```python
from build123d import *

# Parameters (mm, degrees)
SKETCH1_W                = 400
SKETCH1_H                = 700
BOSS_EXTRUDE1_DEPTH      = 10
BOSS_EXTRUDE2_DEPTH      = 200
BOSS_EXTRUDE2_DEPTH_BACK = 200
CUT_EXTRUDE3_DEPTH       = 20
CUT_EXTRUDE3_DEPTH_BACK  = 20
CUT_EXTRUDE4_DEPTH       = 20
CUT_EXTRUDE4_DEPTH_BACK  = 20
CUT_EXTRUDE5_DEPTH       = 20
CUT_EXTRUDE5_DEPTH_BACK  = 20
SHELL3_START             = -189.5
SHELL3_DEPTH             = 379
SHELL3_START_2           = -124.5
SHELL3_2_DEPTH           = 94
SHELL3_START_3           = 30.5
SHELL3_3_DEPTH           = 94
SHELL3_4_DEPTH           = 4
SHELL3_START_4           = 185.5
SHELL3_5_DEPTH           = 4
SHELL3_START_5           = -30.5
SHELL3_6_DEPTH           = 61
FILLET1_R                = 100


# Read off the part's stored shape, not the designer's step: Shell3
with BuildPart() as part:
    # Sketch1 → Boss-Extrude1 (new body)
    with BuildSketch(Plane(origin=(0, 0, 0), x_dir=(1, 0, 0), z_dir=(0, 1, 0))):
        with Locations((0, 350)):
            Rectangle(SKETCH1_W, SKETCH1_H)
    extrude(amount=BOSS_EXTRUDE1_DEPTH)

    # Sketch2 → Boss-Extrude2 (add, two sides: drawn at the far end of the back side and taken through both)
    with BuildSketch(Plane(origin=(0, 0, 0), x_dir=(0, 0, -1), z_dir=(1, 0, 0)).offset(-BOSS_EXTRUDE2_DEPTH_BACK)):
        Polygon((0, 0), (0, 24.464411704), (101.405231438, 51.629278733), (207.601036066, 80.077464993), (207.601036066, 0), align=None)
    extrude(amount=BOSS_EXTRUDE2_DEPTH + BOSS_EXTRUDE2_DEPTH_BACK)

    # Sketch5 → Cut-Extrude3 (cut, two sides: drawn at the far end of the back side and taken through both)
    with BuildSketch(Plane(origin=(0, 0, 0), x_dir=(0, 0, -1), z_dir=(1, 0, 0)).offset(-CUT_EXTRUDE3_DEPTH_BACK)):
        with BuildLine():
            Line((207.651134237, 88.230641516), (207.651134237, 10))
            ThreePointArc((207.651134237, 10), (195.644591457, 43.3333125), (173.411266827, 70.918563406))
            Line((173.411266827, 70.918563406), (207.651134237, 88.230641516))
        make_face()
    extrude(amount=CUT_EXTRUDE3_DEPTH + CUT_EXTRUDE3_DEPTH_BACK, mode=Mode.SUBTRACT)

    # Sketch7 → Cut-Extrude4 (cut, two sides: drawn at the far end of the back side and taken through both)
    with BuildSketch(Plane(origin=(155, 0, 0), x_dir=(0, 0, -1), z_dir=(1, 0, 0)).offset(-CUT_EXTRUDE4_DEPTH_BACK)):
        with BuildLine():
            Line((207.601036066, 80.077464993), (207.601036066, 10))
            ThreePointArc((207.601036066, 10), (195.617643187, 43.328041458), (173.411266827, 70.918563406))
            Line((173.411266827, 70.918563406), (164.696313807, 94.748714882))
            Line((164.696313807, 94.748714882), (211.114914406, 101.759857681))
            Line((211.114914406, 101.759857681), (207.601036066, 80.077464993))
        make_face()
    extrude(amount=CUT_EXTRUDE4_DEPTH + CUT_EXTRUDE4_DEPTH_BACK, mode=Mode.SUBTRACT)

    # Sketch8 → Cut-Extrude5 (cut, two sides: drawn at the far end of the back side and taken through both)
    with BuildSketch(Plane(origin=(-155, 0, 0), x_dir=(0, 0, -1), z_dir=(1, 0, 0)).offset(-CUT_EXTRUDE5_DEPTH_BACK)):
        with BuildLine():
            Line((207.601036066, 10), (207.601036066, 80.077464993))
            Line((207.601036066, 80.077464993), (173.411266827, 70.918563406))
            ThreePointArc((173.411266827, 70.918563406), (195.617643187, 43.328041458), (207.601036066, 10))
        make_face()
    extrude(amount=CUT_EXTRUDE5_DEPTH + CUT_EXTRUDE5_DEPTH_BACK, mode=Mode.SUBTRACT)

    # Shell3 outline → Shell3 (cut)
    with BuildSketch(Plane.YZ.offset(SHELL3_START)):
        with BuildLine():
            Line((10.5, -10.5), (10.5, -196.809675626))
            ThreePointArc((10.5, -196.809675626), (36.812126695, -187.219283255), (59.262427205, -170.477489921))
            Line((59.262427205, -170.477489921), (16.406973107, -10.5))
            Line((16.406973107, -10.5), (10.5, -10.5))
        make_face()
    extrude(amount=SHELL3_DEPTH, mode=Mode.SUBTRACT)

    # Shell3 2 outline → Shell3 2 (cut)
    with BuildSketch(Plane.YZ.offset(SHELL3_START_2)):
        with BuildLine():
            Line((10.5, -207.601036066), (69.207241495, -207.601036066))
            Line((69.207241495, -207.601036066), (59.262427205, -170.477489921))
            ThreePointArc((59.262427205, -170.477489921), (36.812126695, -187.219283255), (10.5, -196.809675626))
            Line((10.5, -196.809675626), (10.5, -207.601036066))
        make_face()
    extrude(amount=SHELL3_2_DEPTH, mode=Mode.SUBTRACT)

    # Shell3 3 outline → Shell3 3 (cut)
    with BuildSketch(Plane.YZ.offset(SHELL3_START_3)):
        with BuildLine():
            Line((10.5, -207.601036066), (69.207241495, -207.601036066))
            Line((69.207241495, -207.601036066), (59.262427205, -170.477489921))
            ThreePointArc((59.262427205, -170.477489921), (36.812126695, -187.219283255), (10.5, -196.809675626))
            Line((10.5, -196.809675626), (10.5, -207.601036066))
        make_face()
    extrude(amount=SHELL3_3_DEPTH, mode=Mode.SUBTRACT)

    # Shell3 4 outline → Shell3 4 (cut)
    with BuildSketch(Plane.YZ.offset(SHELL3_START)):
        with BuildLine():
            Line((10.5, -197.101036066), (66.394456595, -197.101036066))
            Line((66.394456595, -197.101036066), (59.262427205, -170.477489921))
            ThreePointArc((59.262427205, -170.477489921), (36.812126695, -187.219283255), (10.5, -196.809675626))
            Line((10.5, -196.809675626), (10.5, -197.101036066))
        make_face()
    extrude(amount=SHELL3_4_DEPTH, mode=Mode.SUBTRACT)

    # Shell3 5 outline → Shell3 5 (cut)
    with BuildSketch(Plane.YZ.offset(SHELL3_START_4)):
        with BuildLine():
            Line((10.5, -197.101036066), (66.394456595, -197.101036066))
            Line((66.394456595, -197.101036066), (59.262427205, -170.477489921))
            ThreePointArc((59.262427205, -170.477489921), (36.812126695, -187.219283255), (10.5, -196.809675626))
            Line((10.5, -196.809675626), (10.5, -197.101036066))
        make_face()
    extrude(amount=SHELL3_5_DEPTH, mode=Mode.SUBTRACT)

    # Shell3 6 outline → Shell3 6 (cut)
    with BuildSketch(Plane.YZ.offset(SHELL3_START_5)):
        with BuildLine():
            Line((10.5, -196.809675626), (10.5, -196.858395835))
            ThreePointArc((10.5, -196.858395835), (36.816809355, -187.247785942), (59.263801063, -170.482618469))
            Line((59.263801063, -170.482618469), (59.262427205, -170.477489921))
            ThreePointArc((59.262427205, -170.477489921), (36.812126695, -187.219283255), (10.5, -196.809675626))
        make_face()
    extrude(amount=SHELL3_6_DEPTH, mode=Mode.SUBTRACT)

    # Fillet1
    # the kernel refuses this fillet: 100 mm, written as the material it takes off along each edge
    with BuildSketch(Plane(origin=(30.5, 10.5, -207.601036066), x_dir=(0, -1.0, -9.585505722497512e-10), z_dir=(1, 0, 0)), Plane(origin=(-124.5, 10.5, -207.601036066), x_dir=(0, -1.0, -9.585505722497512e-10), z_dir=(1, 0, 0))) as fillet1_piece_1:
        with BuildLine():
            CenterArc((99.99999999, -9.987492273), FILLET1_R, 174.26803198, 5.731967965)
            Line((-1e-08, -9.987492177), (0, 0))
            Line((0, 0), (0.5, 0))
        make_face()
    extrude(amount=94, mode=Mode.SUBTRACT)


solid = part.part
```
Can you work these out from the model? Positions are in its coordinate system, mm. A direction names the side the tool comes from. Round coordinates to 2 decimals unless told otherwise and drop trailing zeros. Order: outer loops, then holes, each group sorted by start corner. A loop starts at its lowest first (then second) coordinate and runs counter-clockwise, first axis right, second up. Notation, with made-up numbers: (21.5, -13.5) -> (26.5, -13.5) arc R23 ccw to (26.5, 23.5) -> close; hole circle Ø6 at (36.5, -5). An arc over 180 degrees is marked (long way). Return JSON: item names as keys, results as strings. Group by question number.
1. If we section it at D-D, the plane x = 164.5: Write out the boundary of the cut face in (y, z).
2. Which directions (+Z, -Z, +X, -X, +Y, -Y) give clear straight access to the entire face, cutting with the end or side of a thin tool? Please do faces 1 (the face through (-135, 58, -195)), 2 (the face through (-3, 0, -355)), 3 (the face through (-124.5, 46, -198)), 4 (the face through (185.5, 50, -190)), 5 (the face through (29, 56, -207.601)).
3. We'd pull the mould along X, two halves only. Please class faces 6 (the face through (-155.28, 43.762, -195.373)), 7 (the face through (-20, 53, -198)), 8 (the face through (187, 46, -207.601)), 9 (the face through (-200, 7, -219)): released by +X, released by -X, zero draft, split by the parting line, or undercut.
4. Will these pins go through, and if not, where does the flat tip stop? pin 1 (2 mm diameter, centred on x = -122, z = -539.5, fed in from +Y); pin 2 (12.5 mm diameter, centred on x = 189, y = 35.5, fed in from -Z); pin 3 (8 mm diameter, centred on x = -15.5, y = 40, fed in from -Z).
5. If we section it at C-C, the plane x = 56.5: Write out the boundary of the cut face in (y, z).
6. I need wall thicknesses on line 1 (Y direction, x = 13, z = -291); line 2 (Y direction, x = -98, z = -154.5); line 3 (Y direction, x = -106.5, z = -189). Which ranges of each line are inside material? Lowest first, please. Write a range as [from, to].
Output values:
{
 "1": {"outline": "(0, -700) -> (10, -700) -> (10, -207.6) arc R107 ccw to (70.92, -173.41) -> (24.46, 0) -> (0, 0) -> close; hole (10.5, -196.81) arc R96.5 ccw to (59.26, -170.48) -> (16.41, -10.5) -> (10.5, -10.5) -> close"},
 "2": {"face 1": "-Z, +Y", "face 2": "+Z, -Z, +X, -X, -Y", "face 3": "-Z", "face 4": "none", "face 5": "-Z, +X, -X, +Y"},
 "3": {"face 6": "undercut", "face 7": "undercut", "face 8": "zero draft", "face 9": "released by -X"},
 "4": {"pin 1": "y = 10", "pin 2": "z = -207.6", "pin 3": "z = -199.4"},
 "5": {"outline": "(0, -700) -> (10, -700) -> (10, -207.6) arc R100 ccw to (10.5, -197.61) -> (10.5, -10.5) -> (16.41, -10.5) -> (69.21, -207.6) -> (80.08, -207.6) -> (24.46, 0) -> (0, 0) -> close"},
 "6": {"line 1": "[0, 10]", "line 2": "[0, 10.5], [54.98, 65.85]", "line 3": "[0, 10.5], [64.22, 75.09]"}
}
